For this review, take the finished solid that the model builds, in its own axes (mm). Give positions to 0.01 mm unless a question says otherwise; leave off trailing zeros. Loops run counter-clockwise (first coordinate to the right, second up) from the corner with the lowest first, then second, coordinate; pieces in that order, holes last. Notation, with made-up numbers: M -37,61 L -1,61 A29 cw -1,88 Z; hole C -5,63.5 d1. An arc over 180 degrees is marked long. Use CSV: the item, a comma, the result in double quotes. Start each with the question number.
1. Take a section at B-B, the plane x = 1.75. Write out the cut boundary in (y, z), and give its area (3 significant figures).
2. Insertion check: P1, Ø0.7, axis at y = 4.5, z = 0, coming from the +X side (3 decimals); P2, Ø0.7, axis at y = -1, z = 0, coming from the -X side (3 decimals); P3, Ø0.5, axis at x = 2.5, y = 5.5, coming from the -Z side (3 decimals). Each pin has a flat end and moves straight along its axis. Give the tip position at first contact, or say it passes through.
3. The part is to be moulded in two halves that separate along X. For faces 1 (the face through (4, 2.54, 0)), 2 (the face through (-1.27, 1, 0)), 3 (the face through (5, 1, 1.27)), say which applies: pulls with the +X half, pulls with the -X half, needs draft (parallel to the pull), parting line crosses it, or undercut.
4. To check wall thickness, follow line 1 (X direction, y = 6.25, z = 0.1) (3 decimals); line 2 (Y direction, x = 8, z = 0.7); line 3 (Y direction, x = 6.5, z = 0.95). State the ranges of each line that lie inside material, in increasing order. Write a range as [from, to].
5. Take a section at A-A, the plane y = 7.25. Write out the cut boundary in (x, z) (3 decimals), and give its area (3 significant figures).
from build123d import *
from OCP.BRepFilletAPI import BRepFilletAPI_MakeChamfer

# Parameters (mm, degrees)
CUT_EXTRUDE1_START   = -2.54
CUT_EXTRUDE1_DEPTH   = 2.286
CUT_EXTRUDE1_START_2 = -0.254
CUT_EXTRUDE1_2_DEPTH = 0.254
SKETCH2_W            = 2.032
SKETCH2_H            = 2.54
CUT_EXTRUDE2_DEPTH   = 0.254
CUT_EXTRUDE3_DEPTH   = 0.254
CUT_EXTRUDE4_DEPTH   = 0.254
BOSS_EXTRUDE1_DEPTH  = 0.254
BOSS_EXTRUDE2_DEPTH  = 0.254
SKETCH7_W            = 0.65
SKETCH7_H            = 0.65
BOSS_EXTRUDE3_DEPTH  = 3.302
SKETCH8_W            = 0.65
SKETCH8_H            = 0.65
BOSS_EXTRUDE4_DEPTH  = 3.302
SKETCH9_W            = 0.65
SKETCH9_H            = 0.65
BOSS_EXTRUDE5_DEPTH  = 3.302
SKETCH10_W           = 0.65
SKETCH10_H           = 0.65
BOSS_EXTRUDE6_DEPTH  = 3.302
SKETCH11_W           = 0.65
SKETCH11_H           = 0.65
BOSS_EXTRUDE7_DEPTH  = 6.35
SKETCH12_W           = 0.65
SKETCH12_H           = 0.65
BOSS_EXTRUDE8_DEPTH  = 6.35
SKETCH13_W           = 0.65
SKETCH13_H           = 0.65
BOSS_EXTRUDE9_DEPTH  = 6.35
SKETCH14_W           = 0.65
SKETCH14_H           = 0.65
BOSS_EXTRUDE10_DEPTH = 6.35
CHAMFER1_SIZE        = 0.254
CHAMFER2_SIZE        = 0.2
CHAMFER2_SIZE2       = 0.4


with BuildPart() as part:
    # Cut-Extrude1: read off the stored shape, not the designer's step
    # Cut-Extrude1 outline → Cut-Extrude1 (new body)
    with BuildSketch(Plane.XZ.offset(CUT_EXTRUDE1_START)):
        Polygon((3.556, 1.27), (1.524, 1.27), (1.27, 1.016), (1.016, 1.27), (-1.016, 1.27), (-1.27, 1.016), (-1.27, -1.27), (1.016, -1.27), (1.27, -1.016), (1.524, -1.27), (3.556, -1.27), (3.81, -1.016), (4.064, -1.27), (6.096, -1.27), (6.35, -1.016), (6.604, -1.27), (8.636, -1.27), (8.89, -1.016), (8.89, 1.27), (6.604, 1.27), (6.35, 1.016), (6.096, 1.27), (4.064, 1.27), (3.81, 1.016), align=None)
    extrude(amount=CUT_EXTRUDE1_DEPTH)

    # Cut-Extrude1 2 outline → Cut-Extrude1 2 (add)
    with BuildSketch(Plane.XZ.offset(CUT_EXTRUDE1_START_2)):
        Polygon((1.27, -1.016), (1.524, -1.27), (1.524, 1.27), (1.27, 1.016), (1.016, 1.27), (-1.016, 1.27), (-1.27, 1.016), (-1.27, -1.27), (1.016, -1.27), align=None)
        Polygon((3.556, 1.27), (3.556, -1.27), (3.81, -1.016), (4.064, -1.27), (6.096, -1.27), (6.35, -1.016), (6.604, -1.27), (8.636, -1.27), (8.89, -1.016), (8.89, 1.27), (6.604, 1.27), (6.35, 1.016), (6.096, 1.27), (4.064, 1.27), (3.81, 1.016), align=None)
    extrude(amount=CUT_EXTRUDE1_2_DEPTH)

    # Sketch2 → Cut-Extrude2 (cut)
    with BuildSketch(Plane.XZ):
        with Locations((5.08, 0)):
            Rectangle(SKETCH2_W, SKETCH2_H)
    extrude(amount=-CUT_EXTRUDE2_DEPTH, mode=Mode.SUBTRACT)

    # Sketch3 → Cut-Extrude3 (cut)
    with BuildSketch(Plane.XZ):
        Polygon((-1.27, -1.27), (1.016, -1.27), (1.016, 1.27), (-1.016, 1.27), (-1.27, 1.016), align=None)
    extrude(amount=-CUT_EXTRUDE3_DEPTH, mode=Mode.SUBTRACT)

    # Sketch4 → Cut-Extrude4 (cut)
    with BuildSketch(Plane.XZ):
        Polygon((6.604, -1.27), (8.636, -1.27), (8.89, -1.016), (8.89, 1.27), (6.604, 1.27), align=None)
    extrude(amount=-CUT_EXTRUDE4_DEPTH, mode=Mode.SUBTRACT)

    # Sketch5 → Boss-Extrude1 (add)
    with BuildSketch(Plane.XZ.offset(-0.254)):
        Polygon((-1.27, -1.27), (-1.27, 1.016), (-1.016, 1.27), (-1.016, -1.27), align=None)
    extrude(amount=BOSS_EXTRUDE1_DEPTH)

    # Sketch6 → Boss-Extrude2 (add)
    with BuildSketch(Plane.XZ.offset(-0.254)):
        Polygon((8.89, 1.27), (8.89, -1.016), (8.636, -1.27), (8.636, 1.27), align=None)
    extrude(amount=BOSS_EXTRUDE2_DEPTH)

    # Sketch7 → Boss-Extrude3 (add)
    with BuildSketch(Plane.XZ.offset(-0.254)):
        Rectangle(SKETCH7_W, SKETCH7_H)
    extrude(amount=BOSS_EXTRUDE3_DEPTH)

    # Sketch8 → Boss-Extrude4 (add)
    with BuildSketch(Plane.XZ.offset(-0.254)):
        with Locations((2.54, 0)):
            Rectangle(SKETCH8_W, SKETCH8_H)
    extrude(amount=BOSS_EXTRUDE4_DEPTH)

    # Sketch9 → Boss-Extrude5 (add)
    with BuildSketch(Plane.XZ.offset(-0.254)):
        with Locations((5.08, 0)):
            Rectangle(SKETCH9_W, SKETCH9_H)
    extrude(amount=BOSS_EXTRUDE5_DEPTH)

    # Sketch10 → Boss-Extrude6 (add)
    with BuildSketch(Plane.XZ.offset(-0.254)):
        with Locations((7.62, 0)):
            Rectangle(SKETCH10_W, SKETCH10_H)
    extrude(amount=BOSS_EXTRUDE6_DEPTH)

    # Sketch11 → Boss-Extrude7 (add)
    with BuildSketch(Plane(origin=(0, 2.54, 0), x_dir=(-1, 0, 0), z_dir=(0, 1, 0))):
        Rectangle(SKETCH11_W, SKETCH11_H)
    extrude(amount=BOSS_EXTRUDE7_DEPTH)

    # Sketch12 → Boss-Extrude8 (add)
    with BuildSketch(Plane(origin=(0, 2.54, 0), x_dir=(-1, 0, 0), z_dir=(0, 1, 0))):
        with Locations((-2.54, 0)):
            Rectangle(SKETCH12_W, SKETCH12_H)
    extrude(amount=BOSS_EXTRUDE8_DEPTH)

    # Sketch13 → Boss-Extrude9 (add)
    with BuildSketch(Plane(origin=(0, 2.54, 0), x_dir=(-1, 0, 0), z_dir=(0, 1, 0))):
        with Locations((-5.08, 0)):
            Rectangle(SKETCH13_W, SKETCH13_H)
    extrude(amount=BOSS_EXTRUDE9_DEPTH)

    # Sketch14 → Boss-Extrude10 (add)
    with BuildSketch(Plane(origin=(0, 2.54, 0), x_dir=(-1, 0, 0), z_dir=(0, 1, 0))):
        with Locations((-7.62, 0)):
            Rectangle(SKETCH14_W, SKETCH14_H)
    extrude(amount=BOSS_EXTRUDE10_DEPTH)

    # Chamfer1
    chamfer1_edges = [part.edges().sort_by_distance(p)[0] for p in [
        (-1.27, 1.27, -1.27),
        (8.89, 1.27, 1.27),
    ]]
    chamfer(chamfer1_edges, length=CHAMFER1_SIZE)

    # Chamfer2: one chamfer whose edges measure the first distance from different faces: ONE call of the kernel's chamfer builder (chamfer() names one face for all edges)
    chamfer2_edges_1 = [part.edges().sort_by_distance(p)[0] for p in [
        (-0.325, -3.048, 0),
        (0, -3.048, -0.325),
        (0.325, -3.048, 0),
        (0, -3.048, 0.325),
    ]]
    chamfer2_side_1 = [part.faces().sort_by_distance(p)[0] for p in [
        (0, -3.048, 0),
    ]]
    chamfer2_edges_2 = [part.edges().sort_by_distance(p)[0] for p in [
        (2.54, -3.048, -0.325),
        (2.865, -3.048, 0),
        (2.54, -3.048, 0.325),
        (2.215, -3.048, 0),
    ]]
    chamfer2_side_2 = [part.faces().sort_by_distance(p)[0] for p in [
        (2.54, -3.048, 0),
    ]]
    chamfer2_edges_3 = [part.edges().sort_by_distance(p)[0] for p in [
        (5.08, -3.048, -0.325),
        (5.405, -3.048, 0),
        (5.08, -3.048, 0.325),
        (4.755, -3.048, 0),
    ]]
    chamfer2_side_3 = [part.faces().sort_by_distance(p)[0] for p in [
        (5.08, -3.048, 0),
    ]]
    chamfer2_edges_4 = [part.edges().sort_by_distance(p)[0] for p in [
        (7.62, -3.048, -0.325),
        (7.945, -3.048, 0),
        (7.62, -3.048, 0.325),
        (7.295, -3.048, 0),
    ]]
    chamfer2_side_4 = [part.faces().sort_by_distance(p)[0] for p in [
        (7.62, -3.048, 0),
    ]]
    chamfer2_edges_5 = [part.edges().sort_by_distance(p)[0] for p in [
        (0, 8.89, -0.325),
        (-0.325, 8.89, 0),
        (0, 8.89, 0.325),
        (0.325, 8.89, 0),
    ]]
    chamfer2_side_5 = [part.faces().sort_by_distance(p)[0] for p in [
        (0, 8.89, 0),
    ]]
    chamfer2_edges_6 = [part.edges().sort_by_distance(p)[0] for p in [
        (2.54, 8.89, -0.325),
        (2.215, 8.89, 0),
        (2.54, 8.89, 0.325),
        (2.865, 8.89, 0),
    ]]
    chamfer2_side_6 = [part.faces().sort_by_distance(p)[0] for p in [
        (2.54, 8.89, 0),
    ]]
    chamfer2_edges_7 = [part.edges().sort_by_distance(p)[0] for p in [
        (5.08, 8.89, -0.325),
        (4.755, 8.89, 0),
        (5.08, 8.89, 0.325),
        (5.405, 8.89, 0),
    ]]
    chamfer2_side_7 = [part.faces().sort_by_distance(p)[0] for p in [
        (5.08, 8.89, 0),
    ]]
    chamfer2_edges_8 = [part.edges().sort_by_distance(p)[0] for p in [
        (7.945, 8.89, 0),
        (7.62, 8.89, -0.325),
        (7.295, 8.89, 0),
        (7.62, 8.89, 0.325),
    ]]
    chamfer2_side_8 = [part.faces().sort_by_distance(p)[0] for p in [
        (7.62, 8.89, 0),
    ]]
    chamfer2 = BRepFilletAPI_MakeChamfer(part.part.solid().wrapped)
    for e in chamfer2_edges_1:
        chamfer2.Add(CHAMFER2_SIZE, CHAMFER2_SIZE2, e.wrapped, chamfer2_side_1[0].wrapped)  # the first distance lies on this face
    for e in chamfer2_edges_2:
        chamfer2.Add(CHAMFER2_SIZE, CHAMFER2_SIZE2, e.wrapped, chamfer2_side_2[0].wrapped)  # the first distance lies on this face
    for e in chamfer2_edges_3:
        chamfer2.Add(CHAMFER2_SIZE, CHAMFER2_SIZE2, e.wrapped, chamfer2_side_3[0].wrapped)  # the first distance lies on this face
    for e in chamfer2_edges_4:
        chamfer2.Add(CHAMFER2_SIZE, CHAMFER2_SIZE2, e.wrapped, chamfer2_side_4[0].wrapped)  # the first distance lies on this face
    for e in chamfer2_edges_5:
        chamfer2.Add(CHAMFER2_SIZE, CHAMFER2_SIZE2, e.wrapped, chamfer2_side_5[0].wrapped)  # the first distance lies on this face
    for e in chamfer2_edges_6:
        chamfer2.Add(CHAMFER2_SIZE, CHAMFER2_SIZE2, e.wrapped, chamfer2_side_6[0].wrapped)  # the first distance lies on this face
    for e in chamfer2_edges_7:
        chamfer2.Add(CHAMFER2_SIZE, CHAMFER2_SIZE2, e.wrapped, chamfer2_side_7[0].wrapped)  # the first distance lies on this face
    for e in chamfer2_edges_8:
        chamfer2.Add(CHAMFER2_SIZE, CHAMFER2_SIZE2, e.wrapped, chamfer2_side_8[0].wrapped)  # the first distance lies on this face
    add(Compound.cast(chamfer2.Shape()), mode=Mode.REPLACE)


solid = part.part
Result set:
1,outline,"M 0.25,-1.27 L 2.54,-1.27 L 2.54,1.27 L 0.25,1.27 Z"
1,area,"5.81 mm2"
2,P1,"x = 7.945"
2,P2,"x = -0.325"
2,P3,"z = -0.325"
3,face 1,"undercut"
3,face 2,"pulls with the -X half"
3,face 3,"needs draft"
4,line 1,"[-0.325, 0.325], [2.215, 2.865], [4.755, 5.405], [7.295, 7.945]"
4,line 2,"[0.25, 2.54]"
4,line 3,"[0, 2.54]"
5,outline,"M -0.325,-0.325 L 0.325,-0.325 L 0.325,0.325 L -0.325,0.325 Z; M 2.215,-0.325 L 2.865,-0.325 L 2.865,0.325 L 2.215,0.325 Z; M 4.755,-0.325 L 5.405,-0.325 L 5.405,0.325 L 4.755,0.325 Z; M 7.295,-0.325 L 7.945,-0.325 L 7.945,0.325 L 7.295,0.325 Z"
5,area,"1.69 mm2"
